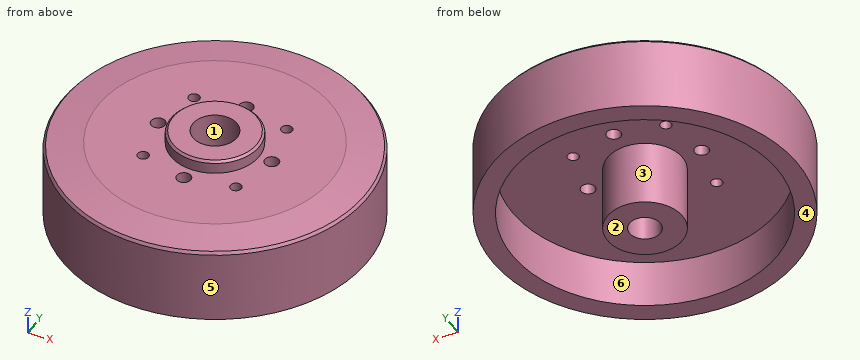
```python
from build123d import *

# Parameters (mm, degrees)
SKETCH2_R                  = 34.5
BOSS_EXTRUDE1_DEPTH        = 18
SKETCH3_R                  = 10
BOSS_EXTRUDE2_DEPTH        = 3
CHAMFER1_SIZE              = 1
CHAMFER1_SIZE2             = 8.144346428
SKETCH4_R                  = 5
CUT_EXTRUDE1_DEPTH         = 21
SKETCH5_R                  = 30
CUT_EXTRUDE2_DEPTH         = 11
M3_TAPPED_HOLE1_D          = 2.5
F_3_2_3_2_DIAMETER_HOLE1_D = 3.2
CHAMFER2_SIZE2             = 0.5
CHAMFER2_SIZE              = 0.574265899
CHAMFER2_EDGE_2_SIZE       = 0.5
SKETCH10_R                 = 8.5
BOSS_EXTRUDE3_DEPTH        = 15
CUT_EXTRUDE3_REACH         = 27
SKETCH11_R                 = 3.5


with BuildPart() as part:
    # Sketch2 → Boss-Extrude1 (new body)
    with BuildSketch(Plane.XY):
        Circle(SKETCH2_R)
    extrude(amount=BOSS_EXTRUDE1_DEPTH)

    # Sketch3 → Boss-Extrude2 (add)
    with BuildSketch(Plane.XY.offset(18)):
        Circle(SKETCH3_R)
    extrude(amount=BOSS_EXTRUDE2_DEPTH)

    # Chamfer1
    chamfer1_edges = [part.edges().sort_by_distance(p)[0] for p in [
        (-34.5, 0, 18),
    ]]
    chamfer1_side = [part.faces().sort_by_distance(p)[0] for p in [
        (-34.5, 0, 9),
    ]]
    chamfer(chamfer1_edges, length=CHAMFER1_SIZE, length2=CHAMFER1_SIZE2, reference=chamfer1_side[0])

    # Sketch4 → Cut-Extrude1 (cut)
    with BuildSketch(Plane.XY.offset(21)):
        Circle(SKETCH4_R)
    extrude(amount=-CUT_EXTRUDE1_DEPTH, mode=Mode.SUBTRACT)

    # Sketch5 → Cut-Extrude2 (cut)
    with BuildSketch(Plane(origin=(0, 0, 0), x_dir=(-1, 0, 0), z_dir=(0, 0, -1))):
        Circle(SKETCH5_R)
    extrude(amount=-CUT_EXTRUDE2_DEPTH, mode=Mode.SUBTRACT)

    # M3 Tapped Hole1 (through all)
    with Locations(Plane.XY.offset(18)):
        with Locations((10.606601718, 10.606601718), (10.606601718, -10.606601718), (-10.606601718, -10.606601718), (-10.606601718, 10.606601718)):
            Hole(M3_TAPPED_HOLE1_D / 2)

    # Ø3.2 (3.2) Diameter Hole1 (through all)
    with Locations(Plane.XY.offset(18)):
        with Locations((13, 0), (-13, 0), (0, 13), (0, -13)):
            Hole(F_3_2_3_2_DIAMETER_HOLE1_D / 2)

    # Chamfer2
    chamfer2_edges = [part.edges().sort_by_distance(p)[0] for p in [
        (-34.5, 0, 17),
    ]]
    chamfer(chamfer2_edges, length=CHAMFER2_SIZE, length2=CHAMFER2_SIZE2)

    # Chamfer2 edge 2
    chamfer2_edge_2_edges = [part.edges().sort_by_distance(p)[0] for p in [
        (-10, 0, 21),
    ]]
    chamfer(chamfer2_edge_2_edges, length=CHAMFER2_EDGE_2_SIZE)

    # Sketch10 → Boss-Extrude3 (add)
    with BuildSketch(Plane(origin=(0, 0, 11), x_dir=(-1, 0, 0), z_dir=(0, 0, -1))):
        Circle(SKETCH10_R)
    extrude(amount=BOSS_EXTRUDE3_DEPTH)

    # Sketch11 → Cut-Extrude3 (cut, up to next)
    with BuildSketch(Plane(origin=(0, 0, -4), x_dir=(-1, 0, 0), z_dir=(0, 0, -1)), mode=Mode.PRIVATE) as cut_extrude3_sk1:
        Circle(SKETCH11_R)
    cut_extrude3_tool1 = extrude(cut_extrude3_sk1.sketch, amount=-CUT_EXTRUDE3_REACH, mode=Mode.PRIVATE) & part.part
    add(cut_extrude3_tool1.solids().sort_by_distance((0, 0, -4))[0], mode=Mode.SUBTRACT)


solid = part.part
```
Can you work these out from the model? Positions are in its coordinate system, mm. Face numbers are marked on the shaded views. A direction names the side the tool comes from. Coordinates: 2 decimals unless noted, no trailing zeros. Loops run counter-clockwise (first coordinate to the right, second up) from the corner with the lowest first, then second, coordinate; pieces in that order, holes last.
1) Imagine slicing it at A-A on z = 6. List the corners of the cut face in (x, y) for me.
2) Imagine slicing it at B-B on z = 13.5. State how many separate pieces and enclosed holes the cut face has, plus the area to 3 significant figures.
3) I need wall thicknesses on probe 1 along Y at (x, z) = (0, 13.5); probe 2 along Y at (x, z) = (-5, 7.5); probe 3 along Y at (x, z) = (4.5, 8.5). Which ranges of each line are inside material? Lowest first, please.
4) Thinking about a two-plate mould opening in Y: for the marked faces 4, 5 and 6, which applies, pulls with the +Y half, pulls with the -Y half, needs draft (parallel to the pull), parting line crosses it, or undercut?
5) Which directions (+Z, -Z, +X, -X, +Y, -Y) give clear straight access to the entire face, cutting with the end or side of a thin tool? Please do the marked faces 1, 2 and 3.
6) For pin 1 (1 mm diameter, centred on y = -8, z = 0.5, fed in from -X); pin 2 (3 mm diameter, centred on x = -0.5, y = 2.5, fed in from +Z); pin 3 (10 mm diameter, centred on x = -13.5, z = 18.5, fed in from -Y), each with a flat end and sliding along its axis, tell me the tip position at first contact or that it passes through.
Completed:
1. outline: circle Ø69 at (0, 0); circle Ø17 at (0, 0); hole circle Ø60 at (0, 0); hole circle Ø7 at (0, 0)
2. separate pieces: 1
2. enclosed holes: 9
2. area: 3,610 mm2
3. probe 1: y = -34.5 to -14.6, -11.4 to -5, 5 to 11.4, 14.6 to 34.5
3. probe 2: y = -34.14 to -29.58, -6.87 to 6.87, 29.58 to 34.14
3. probe 3: y = -34.21 to -29.66, -7.21 to 7.21, 29.66 to 34.21
4. face 4: needs draft
4. face 5: parting line crosses it
4. face 6: undercut
5. face 1: +Z
5. face 2: -Z, +X, -X, +Y, -Y
5. face 3: -Z
6. pin 1: stops at x = -33.67
6. pin 2: stops at z = 11
6. pin 3: stops at y = -33.32
